Read the model definition and answer for the solid it produces. Units are mm, in the model's axes. A direction names the side the tool comes from. Give positions to 0.01 mm unless a question says otherwise; leave off trailing zeros. Write each loop counter-clockwise with the first axis right and the second up, starting at its lowest first coordinate (ties: lowest second). Pieces come first, ordered by that corner, then holes.
```python
from build123d import *

# Parameters (mm, degrees)
BOSS_EXTRUDE1_DEPTH = 3.175
SKETCH4_R           = 2.54
CUT_EXTRUDE3_DEPTH  = 4.175
FILLET1_R           = 5.08
FILLET2_R           = 5.08


with BuildPart() as part:
    # Sketch1 → Boss-Extrude1 (new body)
    with BuildSketch(Plane.XY):
        Polygon((-38.1, 50.8), (-25.4, 50.8), (-25.4, 12.7), (25.4, 12.7), (25.4, 50.8), (38.1, 50.8), (38.1, -50.8), (25.4, -50.8), (25.4, -12.7), (-25.4, -12.7), (-25.4, -50.8), (-38.1, -50.8), align=None)
    extrude(amount=BOSS_EXTRUDE1_DEPTH)

    # Sketch4 → Cut-Extrude3 (cut, through all)
    with BuildSketch(Plane.XY.offset(3.175)):
        with Locations((-31.75, 44.45)):
            Circle(SKETCH4_R)
        with Locations((-31.75, 6.35)):
            Circle(SKETCH4_R)
        with Locations((31.75, 6.35)):
            Circle(SKETCH4_R)
        with Locations((31.75, 44.45)):
            Circle(SKETCH4_R)
        with Locations((-31.75, -6.35)):
            Circle(SKETCH4_R)
        with Locations((31.75, -6.35)):
            Circle(SKETCH4_R)
        with Locations((31.75, -44.45)):
            Circle(SKETCH4_R)
        with Locations((-31.75, -44.45)):
            Circle(SKETCH4_R)
    extrude(amount=-CUT_EXTRUDE3_DEPTH, mode=Mode.SUBTRACT)

    # Fillet1
    fillet1_edges = [part.edges().sort_by_distance(p)[0] for p in [
        (25.4, -12.7, 1.5875),
        (-25.4, -12.7, 1.5875),
        (-25.4, 12.7, 1.5875),
        (25.4, 12.7, 1.5875),
    ]]
    fillet(fillet1_edges, radius=FILLET1_R)

    # Fillet2
    fillet2_edges = [part.edges().sort_by_distance(p)[0] for p in [
        (38.1, 50.8, 1.5875),
        (38.1, -50.8, 1.5875),
        (25.4, -50.8, 1.5875),
        (-25.4, -50.8, 1.5875),
        (-38.1, -50.8, 1.5875),
        (-38.1, 50.8, 1.5875),
        (-25.4, 50.8, 1.5875),
        (25.4, 50.8, 1.5875),
    ]]
    fillet(fillet2_edges, radius=FILLET2_R)


solid = part.part
```
Item 1: Each of these flat-tipped pins is pushed along its axis until it touches: pin 1 Ø1 at (x, z) = (7, 2) entering from -Y; pin 2 Ø6.5 at (x, y) = (-31.75, -6.35) entering from +Z (3 decimals); pin 3 Ø12 at (x, y) = (16, 27) entering from +Z. Where does it stop, or does it pass through?
Result set:
pin 1: stops at y = -12.7
pin 2: stops at z = 3.175
pin 3: passes through
Item 2: Section B-B (y = 44.45) is taken. Write down the section's boundary in (x, z) (3 decimals), and give its area (3 significant figures).
Result set:
outline: (-38.1, 0) - (-34.29, 0) - (-34.29, 3.175) - (-38.1, 3.175) - close; (-29.21, 0) - (-25.4, 0) - (-25.4, 3.175) - (-29.21, 3.175) - close; (25.4, 0) - (29.21, 0) - (29.21, 3.175) - (25.4, 3.175) - close; (34.29, 0) - (38.1, 0) - (38.1, 3.175) - (34.29, 3.175) - close
area: 48.4 mm2
Item 3: Find the intervals of material crossed by line 1 along Y through (x, z) = (31.75, 1.8); line 2 along X through (y, z) = (33.5, 2.05); line 3 along Y through (x, z) = (-32.5, 1.75), in increasing order.
Result set:
line 1: y = -50.8 to -46.99, -41.91 to -8.89, -3.81 to 3.81, 8.89 to 41.91, 46.99 to 50.8
line 2: x = -38.1 to -25.4, 25.4 to 38.1
line 3: y = -50.8 to -46.88, -42.02 to -8.78, -3.92 to 3.92, 8.78 to 42.02, 46.88 to 50.8
Item 4: Section D-D (x = -31.75) is taken. Write down the section's boundary in (y, z) (3 decimals), and give its area (3 significant figures).
Result set:
outline: (-50.8, 0) - (-46.99, 0) - (-46.99, 3.175) - (-50.8, 3.175) - close; (-41.91, 0) - (-8.89, 0) - (-8.89, 3.175) - (-41.91, 3.175) - close; (-3.81, 0) - (3.81, 0) - (3.81, 3.175) - (-3.81, 3.175) - close; (8.89, 0) - (41.91, 0) - (41.91, 3.175) - (8.89, 3.175) - close; (46.99, 0) - (50.8, 0) - (50.8, 3.175) - (46.99, 3.175) - close
area: 258 mm2
Item 5: Determine the mould class of faces 1 (the cylindrical face through (-23.951, 14.228, 1.61)), 2 (the flat face through (-38.1, -1, 2)), 3 (the cylindrical face through (31.42, 46.97, 1.61)), 4 (the flat face through (-32, -50.8, 2)) for opening direction Y: pulls with the +Y half, pulls with the -Y half, needs draft (parallel to the pull), parting line crosses it, or undercut.
Result set:
face 1: pulls with the +Y half
face 2: needs draft
face 3: undercut
face 4: pulls with the -Y half
Item 6: Section C-C (z = 2.05) is taken. Give the number of separate pieces and of enclosed holes in the cut face, and give its area (3 significant figures).
Result set:
separate pieces: 1
enclosed holes: 8
area: 3,690 mm2
Item 7: Section A-A (y = -36) is taken. Write down the section's boundary in (x, z) (3 decimals).
Result set:
outline: (-38.1, 0) - (-25.4, 0) - (-25.4, 3.175) - (-38.1, 3.175) - close; (25.4, 0) - (38.1, 0) - (38.1, 3.175) - (25.4, 3.175) - close
Item 8: Which of the six approach directions +Z, -Z, +X, -X, +Y, -Y give full straight-line access (tool end or side, diameter ignored) to faces 5 (the cylindrical face through (26.928, -49.351, 1.61)), 6 (the cylindrical face through (-33.766, -7.896, 1.61)), 7 (the flat face through (25.4, 32, 2))?
Result set:
face 5: +Z, -Z, -Y
face 6: +Z, -Z
face 7: +Z, -Z, +Y
